from build123d import *

# Parameters (mm, degrees)
SKICA1_W                = 50
SKICA1_H                = 20
P_IDAT_VYSUNUT_M1_DEPTH = 150
SKO_EPINA1_T            = -2


with BuildPart() as part:
    # Skica1 → Přidat vysunutím1 (new body)
    with BuildSketch(Plane.XY):
        with Locations((25, 10)):
            Rectangle(SKICA1_W, SKICA1_H)
    extrude(amount=P_IDAT_VYSUNUT_M1_DEPTH)

    # Skořepina1
    sko_epina1_openings = [part.faces().sort_by_distance(p)[0] for p in [
        (25, 10, 150),
        (25, 10, 0),
    ]]
    offset(amount=SKO_EPINA1_T, openings=sko_epina1_openings, kind=Kind.INTERSECTION)


solid = part.part
The listing builds one solid part. Answer for the finished solid, in the listing's coordinates (mm). A direction names the side the tool comes from. Give positions to 0.01 mm unless a question says otherwise; leave off trailing zeros. Write each loop counter-clockwise with the first axis right and the second up, starting at its lowest first coordinate (ties: lowest second). Pieces come first, ordered by that corner, then holes. Notation, with made-up numbers: (43, 78.25) -> (71, 78.25) arc R8 ccw to (71, 93.25) -> close; hole circle Ø4 at (-31.5, 26.25). An arc over 180 degrees is marked (long way). Use a Markdown table: item, result.
(1) Find the intervals of material crossed by probe 1 along Y at (x, z) = (4.5, 27.5); probe 2 along X at (y, z) = (9.75, 91.5), in increasing order. Write a range as from..to.
Return value:
| item | result |
|---|---|
| probe 1 | 0..2, 18..20 |
| probe 2 | 0..2, 48..50 |
(2) Section A-A, the plane y = 14.5 is taken. Determine the outline of the cut face in (x, z).
Return value:
| item | result |
|---|---|
| outline | (0, 0) -> (2, 0) -> (2, 150) -> (0, 150) -> close; (48, 0) -> (50, 0) -> (50, 150) -> (48, 150) -> close |
(3) Determine the mould class of faces 1 (the flat face through (48, 10, 74)), 2 (the flat face through (25, 0, 74)), 3 (the flat face through (50, 10, 74)) for opening direction X: released by +X, released by -X, zero draft, split by the parting line, or undercut.
Return value:
| item | result |
|---|---|
| face 1 | undercut |
| face 2 | zero draft |
| face 3 | released by +X |
(4) A flat-ended cylindrical pin translates along its axis: P1, Ø8, axis at x = 8.5, y = 11.5, coming from the -Z side. Find the tip coordinate at first contact, or state that the pin passes through.
Return value:
| item | result |
|---|---|
| P1 | through |
(5) For faces 4 (the flat face through (24.9, 18.2, 150)), 5 (the flat face through (2, 10, 74)), determine the directions among +Z, -Z, +X, -X, +Y, -Y from which every point of the face is accessible in a straight line to the end or side of a thin tool.
Return value:
| item | result |
|---|---|
| face 4 | +Z, +X, -X, +Y, -Y |
| face 5 | +Z, -Z |
(6) Section B-B, the plane z = 88 is taken. Determine the outline of the cut face in (x, y).
Return value:
| item | result |
|---|---|
| outline | (0, 0) -> (50, 0) -> (50, 20) -> (0, 20) -> close; hole (2, 2) -> (48, 2) -> (48, 18) -> (2, 18) -> close |
(7) Section C-C, the plane x = 37 is taken. Determine the outline of the cut face in (y, z), then the cut area to 3 significant figures.
Return value:
| item | result |
|---|---|
| outline | (0, 0) -> (2, 0) -> (2, 150) -> (0, 150) -> close; (18, 0) -> (20, 0) -> (20, 150) -> (18, 150) -> close |
| area | 600 mm2 |
